Input: part model. Units: mm. Frame: model coordinates. A direction names the side the tool comes from. Coordinates: 2 decimals unless noted, no trailing zeros. Write each loop counter-clockwise with the first axis right and the second up, starting at its lowest first coordinate (ties: lowest second). Pieces come first, ordered by that corner, then holes. Notation, with made-up numbers: M -39,-10 L -17,-10 A15 ccw -17,17 Z; hole C 68.25,50.25 d10. An arc over 180 degrees is marked long. Use CSV: the item, a comma, the result in double quotes.
```python
from build123d import *

# Parameters (mm, degrees)
F0_W     = 90
F0_H     = 41.77
F1_DEPTH = 6
F3_DEPTH = 44.9
F4_W     = 90
F4_H     = 12
F4_R     = 5
F5_DEPTH = 15
F6_R     = 3
F7_R     = 1.7
F8_DEPTH = 20


with BuildPart() as f1:
    # F0 (on Front) → F1 (new body, symmetric)
    with BuildSketch(Plane.XZ):
        Rectangle(F0_W, F0_H)
    extrude(amount=F1_DEPTH, both=True)

    # F2 (on face) → F3 (join)
    with BuildSketch(Plane.XY.offset(20.885)):
        with BuildLine():
            Line((-28, 0), (-23, 0))
            ThreePointArc((-23, 0), (-28, 5), (-33, 0))
            Line((-33, 0), (-28, 0))
        make_face()
        with BuildLine():
            ThreePointArc((-33, 0), (-28, -5), (-23, 0))
            Line((-23, 0), (-28, 0))
            Line((-28, 0), (-33, 0))
        make_face()
        with BuildLine():
            Line((-5, 0), (0, 0))
            Line((0, 0), (5, 0))
            ThreePointArc((5, 0), (0, 5), (-5, 0))
        make_face()
        with BuildLine():
            Line((5, 0), (0, 0))
            Line((0, 0), (-5, 0))
            ThreePointArc((-5, 0), (0, -5), (5, 0))
        make_face()
        with BuildLine():
            ThreePointArc((33, 0), (28, 5), (23, 0))
            ThreePointArc((23, 0), (28, -5), (33, 0))
        make_face()
    extrude(amount=F3_DEPTH)

    # F4 (on face) → F5 (join)
    with BuildSketch(Plane.XY.offset(65.785)):
        Rectangle(F4_W, F4_H)
        with Locations((-28, 0)):
            Circle(F4_R, mode=Mode.SUBTRACT)
        with Locations((-28, 0)):
            Circle(F4_R)
    extrude(amount=F5_DEPTH)

    # F6
    f6_edges = [f1.edges().sort_by_distance(p)[0] for p in [
        (45, -6, 0),
        (45, 6, 0),
        (-45, -6, 0),
        (-45, 6, 0),
        (-45, 6, 73.285),
        (-45, -6, 73.285),
        (45, -6, 73.285),
        (45, 6, 73.285),
    ]]
    fillet(f6_edges, radius=F6_R)

    # F7 (on face) → F8 (cut)
    with BuildSketch(Plane(origin=(0, 0, 65.785), x_dir=(1, 0, 0), z_dir=(0, 0, -1))):
        with Locations((-28, 0)):
            Circle(F7_R)
        Circle(F7_R)
        with Locations((28, 0)):
            Circle(F7_R)
    extrude(amount=-F8_DEPTH, mode=Mode.SUBTRACT)


solid = f1.part
```
1. Section D-D (z = 62). Return loops of the section in (x, y), then the cut area to 3 significant figures.
Resolved:
outline,"C -28,0 d10; C 0,0 d10; C 28,0 d10"
area,"236 mm^2"
2. Section A-A (x = 20.5). Return loops of the section in (y, z) (3 decimals), then the cut area to 3 significant figures.
Resolved:
outline,"M -6,-20.885 L 6,-20.885 L 6,20.885 L -6,20.885 Z; M -6,65.785 L 6,65.785 L 6,80.785 L -6,80.785 Z"
area,"681 mm^2"
3. Access query for faces 4 (the cylindrical face through (-0.37, 1.66, 73.18)), 5 (the cylindrical face through (-44.14, 5.1, 73.39)), 6 (the cylindrical face through (-23, 0, 43)). Directions: +Z, -Z, +X, -X, +Y, -Y. A direction counts if a zero-diameter tool reaches every point of the face in a straight line with its end or side. Return the directions, or none.
Resolved:
face 4,"+Z"
face 5,"+Z, -Z, -X, +Y"
face 6,"none"
4. Section B-B (y = 0). State how many separate pieces and enclosed holes the cut face has, then the cut area to 3 significant figures.
Resolved:
separate pieces,"1"
enclosed holes,"2"
area,"6,300 mm^2"
5. Mould query, pull axis Z, two halves, no side actions, for faces 1 (the flat face through (-1, 0, -20.885)), 2 (the cylindrical face through (4, 3, 43)), 3 (the cylindrical face through (44.1, 5.14, 0.29)). Classes: pulls with the +Z half, pulls with the -Z half, needs draft (parallel to the pull), parting line crosses it, or undercut.
Resolved:
face 1,"pulls with the -Z half"
face 2,"undercut"
face 3,"needs draft"
6. Material intervals for line 1 (Z direction, x = -40.5, y = 4.25) (3 decimals); line 2 (X direction, y = 0, z = 77.25); line 3 (Y direction, x = -28, z = 75), sorted ascending. Write a range as [from, to].
Resolved:
line 1,"z = [-20.885, 20.885], [65.785, 80.785]"
line 2,"x = [-45, -29.7], [-26.3, -1.7], [1.7, 26.3], [29.7, 45]"
line 3,"y = [-6, -1.7], [1.7, 6]"
7. Contact query for flat-ended pins moving along their axis: pin 1 Ø1 at (x, y) = (27.5, 0.5) entering from +Z (3 decimals); pin 2 Ø2 at (y, z) = (-0.5, 32) entering from +X; pin 3 Ø4 at (y, z) = (-4.5, 23) entering from +X. Output: stop coordinate, or through.
Resolved:
pin 1,"stops at z = 65.785"
pin 2,"stops at x = 33"
pin 3,"stops at x = 32.33"
8. Section C-C (x = -28). Return loops of the section in (y, z) (3 decimals).
Resolved:
outline,"M -6,-20.885 L 6,-20.885 L 6,20.885 L 5,20.885 L 5,65.785 L 6,65.785 L 6,80.785 L 1.7,80.785 L 1.7,65.785 L -1.7,65.785 L -1.7,80.785 L -6,80.785 L -6,65.785 L -5,65.785 L -5,20.885 L -6,20.885 Z"
